Verification items for the finished model (mm, model axes). Coordinates: 2 decimals unless noted, no trailing zeros. Loops run counter-clockwise (first coordinate to the right, second up) from the corner with the lowest first, then second, coordinate; pieces in that order, holes last. Notation, with made-up numbers: M -26.75,-29.5 L 5.25,-29.5 A15 cw 5.25,-15.5 Z; hole C 18,8 d1. An arc over 180 degrees is marked long. Write item = value, one per line. Start each with the question number.
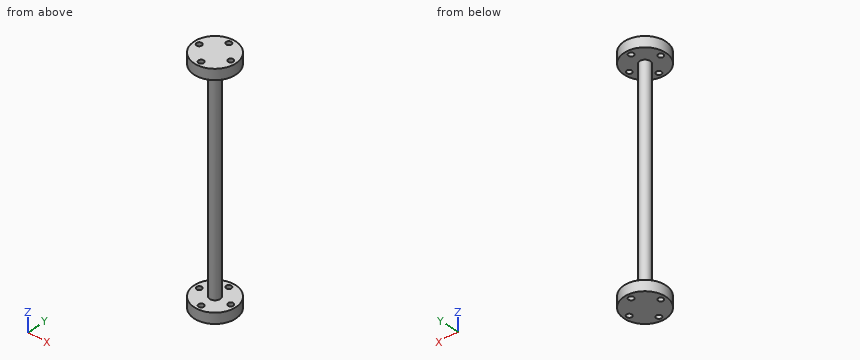
```python
from build123d import *

# Parameters (mm, degrees)
SKETCH1_R                = 5
BOSS_EXTRUDE1_DEPTH      = 105
BOSS_EXTRUDE1_DEPTH_BACK = 100
SKETCH2_R                = 20
SKETCH2_R_2              = 2.5
BOSS_EXTRUDE2_DEPTH      = 10
SKETCH3_R                = 20
SKETCH3_R_2              = 2.5
BOSS_EXTRUDE3_DEPTH      = 10


with BuildPart() as part:
    # Sketch1 → Boss-Extrude1 (new body, two sides)
    with BuildSketch(Plane.XY) as boss_extrude1_sk:
        Circle(SKETCH1_R)
    extrude(amount=BOSS_EXTRUDE1_DEPTH)
    extrude(boss_extrude1_sk.sketch, amount=-BOSS_EXTRUDE1_DEPTH_BACK)

    # Sketch2 → Boss-Extrude2 (add)
    with BuildSketch(Plane.XY.offset(105)):
        Circle(SKETCH2_R)
        with Locations((0, 15)):
            Circle(SKETCH2_R_2, mode=Mode.SUBTRACT)
        with Locations((15, 0)):
            Circle(SKETCH2_R_2, mode=Mode.SUBTRACT)
        with Locations((0, -15)):
            Circle(SKETCH2_R_2, mode=Mode.SUBTRACT)
        with Locations((-15, 0)):
            Circle(SKETCH2_R_2, mode=Mode.SUBTRACT)
    extrude(amount=BOSS_EXTRUDE2_DEPTH)

    # Sketch3 → Boss-Extrude3 (add)
    with BuildSketch(Plane(origin=(0, 0, -100), x_dir=(-1, 0, 0), z_dir=(0, 0, -1))):
        Circle(SKETCH3_R)
        with Locations((0, 15)):
            Circle(SKETCH3_R_2, mode=Mode.SUBTRACT)
        with Locations((-15, 0)):
            Circle(SKETCH3_R_2, mode=Mode.SUBTRACT)
        with Locations((0, -15)):
            Circle(SKETCH3_R_2, mode=Mode.SUBTRACT)
        with Locations((15, 0)):
            Circle(SKETCH3_R_2, mode=Mode.SUBTRACT)
    extrude(amount=BOSS_EXTRUDE3_DEPTH)


solid = part.part
```
Q1. Scan lines: L1, parallel to Y at x = 0, z = -106; L2, parallel to Z at x = -14, y = 2.5; L3, parallel to Y at x = -15, z = -104. Record each from-to range of solid material in increasing order. Write a range as [from, to].
Q2. Sectioned sample at A-A on x = 0. Record the cut outline in (y, z), plus the area to 3 significant figures.
Q3. Gauge pin test, flat end, axial feed: pin 1 (10 mm diameter, centred on y = -2.5, z = 51.5, fed in from +X). Record the tip position at first contact, or that the pin passes through.
Q4. Sectioned sample at C-C on y = 15. Record the cut outline in (x, z).
Solutions:
q1.L1 = [-20, -17.5], [-12.5, 12.5], [17.5, 20]
q1.L2 = [-110, -100], [105, 115]
q1.L3 = [-13.23, -2.5], [2.5, 13.23]
q2.outline = M -20,-110 L -17.5,-110 L -17.5,-100 L -20,-100 Z; M -20,105 L -17.5,105 L -17.5,115 L -20,115 Z; M -12.5,-110 L 12.5,-110 L 12.5,-100 L 5,-100 L 5,105 L 12.5,105 L 12.5,115 L -12.5,115 L -12.5,105 L -5,105 L -5,-100 L -12.5,-100 Z; M 17.5,-110 L 20,-110 L 20,-100 L 17.5,-100 Z; M 17.5,105 L 20,105 L 20,115 L 17.5,115 Z
q2.area = 2,650 mm²
q3.pin_1 = 5
q4.outline = M -13.23,-110 L -2.5,-110 L -2.5,-100 L -13.23,-100 Z; M -13.23,105 L -2.5,105 L -2.5,115 L -13.23,115 Z; M 2.5,-110 L 13.23,-110 L 13.23,-100 L 2.5,-100 Z; M 2.5,105 L 13.23,105 L 13.23,115 L 2.5,115 Z
